from build123d import *

# Parameters (mm, degrees)
SKETCH_1_W          = 60
SKETCH_1_H          = 17
EXTRUDE_1_DEPTH     = 1.2
CUT_EXTRUDE_1_REACH = 33.204
SKETCH_4_R          = 3.25
SKETCH_4_W          = 8
SKETCH_4_H          = 3.9
SKETCH_4_W_2        = 16.2
SKETCH_4_H_2        = 6.8
SKETCH_4_H_3        = 2.9
SKETCH_4_W_3        = 6.5
SKETCH_4_H_4        = 3.5
SKETCH_4_W_4        = 9.8
FILLET_2_R          = 1
CHAMFER_1_SIZE      = 0.8
SKETCH_5_W          = 1.5
SKETCH_5_H          = 8
EXTRUDE_2_DEPTH     = 1.2
SKETCH_6_W          = 28.5
SKETCH_6_H          = 1.6
EXTRUDE_3_DEPTH     = 4
FILLET_3_R          = 1
CHAMFER_2_SIZE      = 1
FILLET_4_R          = 2
CHAMFER_5_SIZE      = 0.4
CHAMFER_6_SIZE      = 1.5


with BuildPart() as part:
    # 草图1 → 凸台-拉伸1 (new body)
    with BuildSketch(Plane(origin=(0, 0, 0), x_dir=(1, 0, 0), z_dir=(0, 1, 0))):
        Rectangle(SKETCH_1_W, SKETCH_1_H)
    extrude(amount=EXTRUDE_1_DEPTH)

    # 草图4 → 切除-拉伸1 (cut, up to next)
    with BuildSketch(Plane(origin=(0, 1.2, 0), x_dir=(1, 0, 0), z_dir=(0, 1, 0)), mode=Mode.PRIVATE) as cut_extrude_1_sk1:
        with Locations(Location((22.298485985, 3.98318929, 0), (0, 0, 270))):
            Circle(SKETCH_4_R)
    cut_extrude_1_tool1 = extrude(cut_extrude_1_sk1.sketch, amount=-CUT_EXTRUDE_1_REACH, mode=Mode.PRIVATE) & part.part
    # 草图4 → 切除-拉伸1 (cut, up to next)
    with BuildSketch(Plane(origin=(0, 1.2, 0), x_dir=(1, 0, 0), z_dir=(0, 1, 0)), mode=Mode.PRIVATE) as cut_extrude_1_sk2:
        with Locations((-20.8, 2.85)):
            Rectangle(SKETCH_4_W, SKETCH_4_H)
    cut_extrude_1_tool2 = extrude(cut_extrude_1_sk2.sketch, amount=-CUT_EXTRUDE_1_REACH, mode=Mode.PRIVATE) & part.part
    # 草图4 → 切除-拉伸1 (cut, up to next)
    with BuildSketch(Plane(origin=(0, 1.2, 0), x_dir=(1, 0, 0), z_dir=(0, 1, 0)), mode=Mode.PRIVATE) as cut_extrude_1_sk3:
        with Locations((0.6, 4.3)):
            Rectangle(SKETCH_4_W_2, SKETCH_4_H_2)
    cut_extrude_1_tool3 = extrude(cut_extrude_1_sk3.sketch, amount=-CUT_EXTRUDE_1_REACH, mode=Mode.PRIVATE) & part.part
    # 草图4 → 切除-拉伸1 (cut, up to next)
    with BuildSketch(Plane(origin=(0, 1.2, 0), x_dir=(1, 0, 0), z_dir=(0, 1, 0)), mode=Mode.PRIVATE) as cut_extrude_1_sk4:
        with Locations((21.05, -4.584803861)):
            Rectangle(SKETCH_4_W, SKETCH_4_H_3)
    cut_extrude_1_tool4 = extrude(cut_extrude_1_sk4.sketch, amount=-CUT_EXTRUDE_1_REACH, mode=Mode.PRIVATE) & part.part
    # 草图4 → 切除-拉伸1 (cut, up to next)
    with BuildSketch(Plane(origin=(0, 1.2, 0), x_dir=(1, 0, 0), z_dir=(0, 1, 0)), mode=Mode.PRIVATE) as cut_extrude_1_sk5:
        with Locations((-1.65, -4.884803861)):
            Rectangle(SKETCH_4_W_3, SKETCH_4_H_4)
    cut_extrude_1_tool5 = extrude(cut_extrude_1_sk5.sketch, amount=-CUT_EXTRUDE_1_REACH, mode=Mode.PRIVATE) & part.part
    # 草图4 → 切除-拉伸1 (cut, up to next)
    with BuildSketch(Plane(origin=(0, 1.2, 0), x_dir=(1, 0, 0), z_dir=(0, 1, 0)), mode=Mode.PRIVATE) as cut_extrude_1_sk6:
        with Locations((-10.15, -4.884803861)):
            Rectangle(SKETCH_4_W_3, SKETCH_4_H_4)
    cut_extrude_1_tool6 = extrude(cut_extrude_1_sk6.sketch, amount=-CUT_EXTRUDE_1_REACH, mode=Mode.PRIVATE) & part.part
    # 草图4 → 切除-拉伸1 (cut, up to next)
    with BuildSketch(Plane(origin=(0, 1.2, 0), x_dir=(1, 0, 0), z_dir=(0, 1, 0)), mode=Mode.PRIVATE) as cut_extrude_1_sk7:
        with Locations((-19.9, -5.084803861)):
            Rectangle(SKETCH_4_W_4, SKETCH_4_H)
    cut_extrude_1_tool7 = extrude(cut_extrude_1_sk7.sketch, amount=-CUT_EXTRUDE_1_REACH, mode=Mode.PRIVATE) & part.part
    add(cut_extrude_1_tool1.solids().sort_by_distance((22.298486, 1.2, -3.983189))[0], mode=Mode.SUBTRACT)
    add(cut_extrude_1_tool2.solids().sort_by_distance((-20.8, 1.2, -2.85))[0], mode=Mode.SUBTRACT)
    add(cut_extrude_1_tool3.solids().sort_by_distance((0.6, 1.2, -4.3))[0], mode=Mode.SUBTRACT)
    add(cut_extrude_1_tool4.solids().sort_by_distance((21.05, 1.2, 4.584804))[0], mode=Mode.SUBTRACT)
    add(cut_extrude_1_tool5.solids().sort_by_distance((-1.65, 1.2, 4.884804))[0], mode=Mode.SUBTRACT)
    add(cut_extrude_1_tool6.solids().sort_by_distance((-10.15, 1.2, 4.884804))[0], mode=Mode.SUBTRACT)
    add(cut_extrude_1_tool7.solids().sort_by_distance((-19.9, 1.2, 5.084804))[0], mode=Mode.SUBTRACT)

    # 圆角2
    fillet_2_edges = [part.edges().sort_by_distance(p)[0] for p in [
        (-13.4, 0.6, 6.634803861),
        (-13.4, 0.6, 3.134803861),
        (-6.9, 0.6, 3.134803861),
        (-6.9, 0.6, 6.634803861),
        (-4.9, 0.6, 6.634803861),
        (-4.9, 0.6, 3.134803861),
        (1.6, 0.6, 3.134803861),
        (1.6, 0.6, 6.634803861),
        (17.05, 0.6, 6.034803861),
        (25.05, 0.6, 6.034803861),
        (-7.5, 0.6, -7.7),
        (8.7, 0.6, -7.7),
        (-24.8, 0.6, 7.034803861),
        (-24.8, 0.6, 3.134803861),
        (-15, 0.6, 3.134803861),
        (-15, 0.6, 7.034803861),
        (-24.8, 0.6, -4.8),
        (-16.8, 0.6, -4.8),
    ]]
    fillet(fillet_2_edges, radius=FILLET_2_R)

    # 倒角1
    chamfer_1_edges = [part.edges().sort_by_distance(p)[0] for p in [
        (17.05, 0.6, 3.134803861),
        (25.05, 0.6, 3.134803861),
        (-24.8, 0.6, -0.9),
        (-16.8, 0.6, -0.9),
    ]]
    chamfer(chamfer_1_edges, length=CHAMFER_1_SIZE)

    # 草图5 → 凸台-拉伸2 (add)
    with BuildSketch(Plane.XZ):
        with Locations((-13.15891381, 0.61681071)):
            Rectangle(SKETCH_5_W, SKETCH_5_H)
        with Locations((13.84108619, 0.61681071)):
            Rectangle(SKETCH_5_W, SKETCH_5_H)
    extrude(amount=EXTRUDE_2_DEPTH)

    # 草图6 → 凸台-拉伸3 (add)
    with BuildSketch(Plane.XZ):
        with Locations((0.34108619, 1.3)):
            Rectangle(SKETCH_6_W, SKETCH_6_H)
    extrude(amount=EXTRUDE_3_DEPTH)

    # 圆角3
    fillet_3_edges = [part.edges().sort_by_distance(p)[0] for p in [
        (-13.90891381, -4, 1.3),
        (14.59108619, -4, 1.3),
    ]]
    fillet(fillet_3_edges, radius=FILLET_3_R)

    # 倒角2
    chamfer_2_edges = [part.edges().sort_by_distance(p)[0] for p in [
        (-13.15891381, -1.2, -3.38318929),
        (-13.15891381, -1.2, 4.61681071),
        (13.84108619, -1.2, -3.38318929),
        (13.84108619, -1.2, 4.61681071),
    ]]
    chamfer(chamfer_2_edges, length=CHAMFER_2_SIZE)

    # 圆角4
    fillet_4_edges = [part.edges().sort_by_distance(p)[0] for p in [
        (30, 0.6, 8.5),
        (-30, 0.6, 8.5),
        (-30, 0.6, -8.5),
        (30, 0.6, -8.5),
    ]]
    fillet(fillet_4_edges, radius=FILLET_4_R)

    # 倒角5
    chamfer_5_edges = [part.edges().sort_by_distance(p)[0] for p in [
        (30, 0, 0),
        (0, 0, 8.5),
        (-30, 0, 0),
        (0, 0, -8.5),
        (-29.414213562, 0, -7.914213562),
        (-29.414213562, 0, 7.914213562),
        (29.414213562, 0, -7.914213562),
        (29.414213562, 0, 7.914213562),
    ]]
    chamfer(chamfer_5_edges, length=CHAMFER_5_SIZE)

    # 倒角6
    chamfer_6_edges = [part.edges().sort_by_distance(p)[0] for p in [
        (-7.5, 0.6, -0.9),
        (8.7, 0.6, -0.9),
    ]]
    chamfer(chamfer_6_edges, length=CHAMFER_6_SIZE)


solid = part.part
Build history of the part. All positions in model axes, mm. A direction names the side the tool comes from. Round coordinates to 2 decimals unless told otherwise and drop trailing zeros. Loops run counter-clockwise (first coordinate to the right, second up) from the corner with the lowest first, then second, coordinate; pieces in that order, holes last. Notation, with made-up numbers: (45.25, -27) -> (104.25, -27) arc R27 ccw to (104.25, 0) -> close; hole circle Ø3 at (-2.75, -25). An arc over 180 degrees is marked (long way). Answer in a Markdown table with one row per item.
Item 1: Mould opens along Z. For faces 5 (the flat face through (13.831, -0.693, 4.124)), 6 (the flat face through (13.091, -1, -1)), 7 (the flat face through (-24.8, 1, 5)) say: +Z half, -Z half, draft (parallel to the pull), parting line (faces both ways), or undercut.
Answers below:
| item | result |
|---|---|
| face 5 | +Z half |
| face 6 | draft |
| face 7 | undercut |
Item 2: Saw through at B-B (x = -21). Write the cut outline in (y, z), and give its area (3 significant figures).
Answers below:
| item | result |
|---|---|
| outline | (0, -8.1) -> (0.4, -8.5) -> (1.2, -8.5) -> (1.2, -4.8) -> (0, -4.8) -> close; (0, -0.9) -> (1.2, -0.9) -> (1.2, 3.13) -> (0, 3.13) -> close; (0, 7.03) -> (1.2, 7.03) -> (1.2, 8.5) -> (0.4, 8.5) -> (0, 8.1) -> close |
| area | 10.9 mm² |
Item 3: Saw through at A-A (x = -9.5). Write the cut outline in (y, z).
Answers below:
| item | result |
|---|---|
| outline | (-4, 0.5) -> (0, 0.5) -> (0, -8.1) -> (0.4, -8.5) -> (1.2, -8.5) -> (1.2, 3.13) -> (0, 3.13) -> (0, 2.1) -> (-4, 2.1) -> close; (0, 6.63) -> (1.2, 6.63) -> (1.2, 8.5) -> (0.4, 8.5) -> (0, 8.1) -> close |
Item 4: Which spindle directions (+Z, -Z, +X, -X, +Y, -Y) get a long thin tool onto all of the face, cutting with end or side? Do faces 1 (the flat face through (-12.409, -1, -1)), 2 (the flat face through (-21, 1, -4.8)), 3 (the flat face through (14, -1.2, -1)), 4 (the conical face through (-29.199, 0.114, -7.725)). Say none if no direction does.
Answers below:
| item | result |
|---|---|
| face 1 | -Z, -Y |
| face 2 | +Y, -Y |
| face 3 | -Z, +X, -X, -Y |
| face 4 | -Z, -X, -Y |
Item 5: Saw through at D-D (y = -1.75). Write the cut outline in (x, z), and give its area (3 significant figures).
Answers below:
| item | result |
|---|---|
| outline | (-13.91, 0.5) -> (14.59, 0.5) -> (14.59, 2.1) -> (-13.91, 2.1) -> close |
| area | 45.6 mm² |
Item 6: Saw through at C-C (x = 5). Write the cut outline in (y, z), and give its area (3 significant figures).
Answers below:
| item | result |
|---|---|
| outline | (-4, 0.5) -> (0, 0.5) -> (0, -0.9) -> (1.2, -0.9) -> (1.2, 8.5) -> (0.4, 8.5) -> (0, 8.1) -> (0, 2.1) -> (-4, 2.1) -> close; (0, -8.1) -> (0.4, -8.5) -> (1.2, -8.5) -> (1.2, -7.7) -> (0, -7.7) -> close |
| area | 18.5 mm² |
Item 7: Pin check, flat tips, straight feed: pin 1 (2 mm diameter, centred on y = -1.5, z = -3, fed in from +X); pin 2 (1.5 mm diameter, centred on x = 21, y = -1.5, fed in from -Z); pin 3 (0.8 mm diameter, centred on x = -13, z = 3, fed in from -Y); pin 4 (6 mm diameter, centred on x = -4.5, z = 3, fed in from -Y). Stop position of each tip, or through.
Answers below:
| item | result |
|---|---|
| pin 1 | stops at x = 14.59 |
| pin 2 | passes through |
| pin 3 | stops at y = -1.2 |
| pin 4 | stops at y = -4 |
Item 8: Drill centre lines: L1, parallel to X at y = -2.6, z = 0.75; L2, parallel to Y at x = -11, z = -7.25; L3, parallel to Z at x = 13, y = -0.2. Where is each one in solid material? Low to high. Write a range as [from, to].
Answers below:
| item | result |
|---|---|
| L1 | x = [-13.91, 14.59] |
| L2 | y = [0, 1.2] |
| L3 | z = [0.5, 2.1] |
